Verification items for the finished model (mm, model axes). Face numbers are marked on the shaded views. A direction names the side the tool comes from. Give positions to 0.01 mm unless a question says otherwise; leave off trailing zeros. Loops run counter-clockwise (first coordinate to the right, second up) from the corner with the lowest first, then second, coordinate; pieces in that order, holes last. Notation, with made-up numbers: (-5.5, 76) - (24.5, 76) arc R20 cw to (24.5, 106) - close; hole circle Ø6 at (-5, -12.5). An arc over 180 degrees is marked (long way). One line per question, with ' | ' between items. Start each with the question number.
1. Thickness scan on line 1 along Z through (x, y) = (36, -7); line 2 along X through (y, z) = (12, -22); line 3 along X through (y, z) = (-34, -14.5). Record the ranges inside material, lowest first. Write a range as from..to.
2. Section check C-C, the plane z = -13. Enter the section's corners in (x, y), then the cut area to 3 significant figures.
3. Section check D-D, the plane y = -8.5. Enter the section's corners in (x, z), then the cut area to 3 significant figures.
4. Mould release check, pull along Z, two halves, no side actions. Record for the marked faces 4, 5, 6 and 7: +Z half, -Z half, draft (parallel to the pull), parting line (faces both ways), or undercut.
5. Depth check by flat-ended pin: pin 1 Ø8 at (y, z) = (1.5, -15.5) entering from +X; pin 2 Ø14 at (y, z) = (-27.5, -22) entering from +X; pin 3 Ø12 at (y, z) = (-31.5, -34) entering from -X; pin 4 Ø5 at (x, y) = (26.5, -30) entering from +Z. Enter the tip coordinate at first touch or a pass-through.
6. Tool access check on the marked faces 1, 2 and 3. Record the directions out of +Z, -Z, +X, -X, +Y, -Y that give a thin tool (end or side, any length) a straight path to the whole face; none if there is none.
7. Section check A-A, the plane x = 4. Enter the section's corners in (y, z), then the cut area to 3 significant figures.
8. Section check B-B, the plane y = 18. Enter the section's corners in (x, z), then the cut area to 3 significant figures.
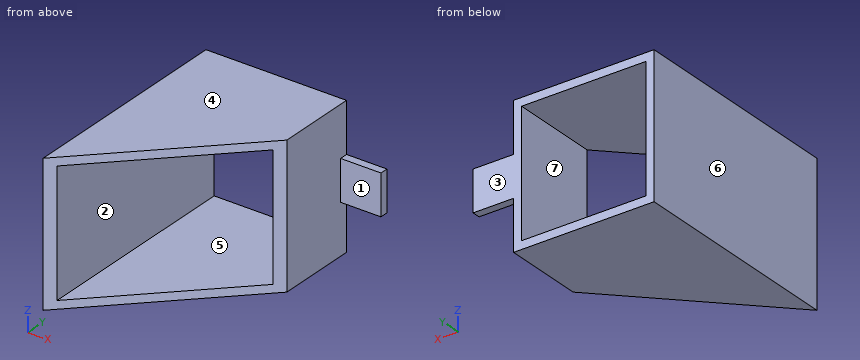
from build123d import *

# Parameters (mm, degrees)
CROQUIS1_W              = 52
CROQUIS1_H              = 52
SALIENTE_EXTRUIR1_DEPTH = 30
SALIENTE_EXTRUIR2_DEPTH = 52
VACIADO4_T              = -3
SALIENTE_EXTRUIR3_DEPTH = 3


with BuildPart() as part:
    # Croquis1 → Saliente-Extruir1 (new body)
    with BuildSketch(Plane(origin=(0, 0, 0), x_dir=(1, 0, 0), z_dir=(0, 1, 0))):
        with Locations((26, 26)):
            Rectangle(CROQUIS1_W, CROQUIS1_H)
    extrude(amount=SALIENTE_EXTRUIR1_DEPTH)

    # Croquis2 → Saliente-Extruir2 (add)
    with BuildSketch(Plane.XY):
        Polygon((0, 0), (0, -52), (52, 0), align=None)
    extrude(amount=-SALIENTE_EXTRUIR2_DEPTH)

    # Vaciado4
    vaciado4_openings = [part.faces().sort_by_distance(p)[0] for p in [
        (26, 30, -26),
        (26, -26, -26),
    ]]
    offset(amount=VACIADO4_T, openings=vaciado4_openings, kind=Kind.INTERSECTION)

    # Croquis3 → Saliente-Extruir3 (add)
    with BuildSketch(Plane(origin=(0, 30, 0), x_dir=(1, 0, 0), z_dir=(0, 1, 0))):
        Polygon((52, 18.5), (67, 18.5), (67, 26), (67, 33.5), (52, 33.5), align=None)
    extrude(amount=-SALIENTE_EXTRUIR3_DEPTH)


solid = part.part
Results list:
1) line 1: -52..-49, -3..0 | line 2: 0..3, 49..52 | line 3: 0..3
2) outline: (0, -52) - (3, -49) - (3, 30) - (0, 30) - close; (49, -3) - (52, 0) - (52, 30) - (49, 30) - close | area: 336 mm²
3) outline: (0, -52) - (43.5, -52) - (43.5, -49) - (3, -49) - (3, -3) - (43.5, -3) - (43.5, 0) - (0, 0) - close | area: 399 mm²
4) face 4: +Z half | face 5: undercut | face 6: draft | face 7: undercut
5) pin 1: x = 52 | pin 2: x = 3 | pin 3: x = 0 | pin 4: through
6) face 1: +Z, -Z, +X, -Y | face 2: +Y, -Y | face 3: +Z, -Z, +X, -X, +Y
7) outline: (-48, -52) - (30, -52) - (30, -49) - (-48, -49) - close; (-48, -3) - (30, -3) - (30, 0) - (-48, 0) - close | area: 468 mm²
8) outline: (0, -52) - (52, -52) - (52, 0) - (0, 0) - close; hole (3, -49) - (49, -49) - (49, -3) - (3, -3) - close | area: 588 mm²
